Verification items for this drawing (mm, ordinates from the low corner). Coordinates: 2 decimals unless noted, no trailing zeros. Write each loop counter-clockwise with the first axis right and the second up, starting at its lowest first coordinate (ties: lowest second). Pieces come first, ordered by that corner, then holes. Notation, with made-up numbers: (-4, -10.75) -> (52, -10.75) arc R16 cw to (52, 0.25) -> close; hole circle Ø4 at (63.5, 49.25). An arc over 180 degrees is marked (long way). Use CSV: the item, a comma, the result in double quotes.
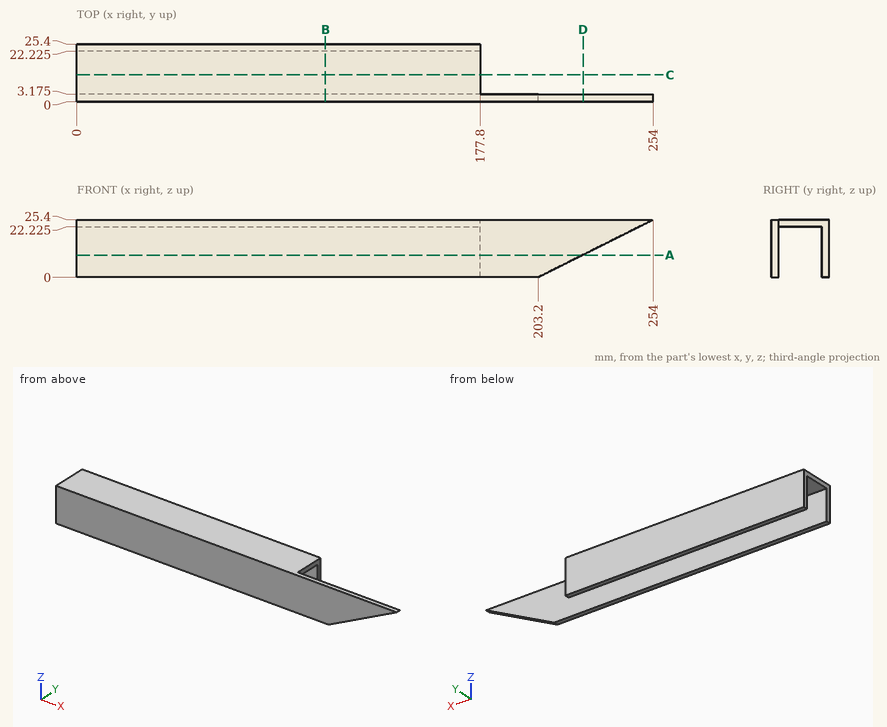
1) Cross-section at D-D (x = 223). Record the boundary of the cut face in (y, z) (3 decimals).
Return value:
outline,"(0, 9.9) -> (3.175, 9.9) -> (3.175, 25.4) -> (0, 25.4) -> close"
2) Cross-section at A-A (z = 9.75). Record the boundary of the cut face in (x, y) (3 decimals).
Return value:
outline,"(0, 0) -> (222.7, 0) -> (222.7, 3.175) -> (0, 3.175) -> close; (0, 22.225) -> (177.8, 22.225) -> (177.8, 25.4) -> (0, 25.4) -> close"
3) Scan lines: L1, parallel to Y at x = 91, z = 8 (3 decimals); L2, parallel to Z at x = 155.5, y = 5.75 (3 decimals); L3, parallel to X at y = 4.75, z = 24. Record each from-to range of solid material in increasing order.
Return value:
L1,"0 to 3.175, 22.225 to 25.4"
L2,"22.225 to 25.4"
L3,"0 to 177.8"
4) Cross-section at C-C (y = 11.75). Record the boundary of the cut face in (x, z) (3 decimals).
Return value:
outline,"(0, 22.225) -> (177.8, 22.225) -> (177.8, 25.4) -> (0, 25.4) -> close"
5) Gauge pin test, flat ends, axial feed: pin 1 (1.5 mm diameter, centred on x = 162, z = 17, fed in from -Y); pin 2 (5 mm diameter, centred on y = 6.5, z = 11.5, fed in from -X). Record the tip position at first contact, or that the pin passes through.
Return value:
pin 1,"y = 0"
pin 2,"through"
6) Cross-section at B-B (x = 109.5). Record the boundary of the cut face in (y, z) (3 decimals).
Return value:
outline,"(0, 0) -> (3.175, 0) -> (3.175, 22.225) -> (22.225, 22.225) -> (22.225, 0) -> (25.4, 0) -> (25.4, 25.4) -> (0, 25.4) -> close"
